Build history of the part. All positions in model axes, mm. A direction names the side the tool comes from. Give positions to 0.01 mm unless a question says otherwise; leave off trailing zeros. Order: outer loops, then holes, each group sorted by start corner. A loop starts at its lowest first (then second) coordinate and runs counter-clockwise, first axis right, second up. Notation, with made-up numbers: (-10, 54.25) - (18, 54.25) arc R26 ccw to (18, 79.25) - close; hole circle Ø11 at (84, 35). An arc over 180 degrees is marked (long way). Write each question's results on one line, items separated by ' | '. Start each with the question number.
1) Cut at B-B on z = 12. List the corners of the cut face in (x, y), plus the area to 3 significant figures.
2) Drop flat-ended pins along their axis: pin 1 Ø6 at (y, z) = (-7, 20) entering from -X; pin 2 Ø6 at (x, y) = (9.5, -5.5) entering from +Z; pin 3 Ø0.7 at (x, z) = (-13, 28) entering from +Y; pin 4 Ø3 at (y, z) = (4, 13) entering from +X. Give the stop position or say it passes through.
3) Drill centre lines: line 1 along Y through (x, z) = (0, 10); line 2 along Z through (x, y) = (11.75, 3.75); line 3 along Z through (x, y) = (12, -7.5). Where is each one in solid material? Low to high. Write a range as from..to.
4) Tool access for faces 1 (the face through (-10.25, 9.09, 29.45)), 2 (the face through (-13, 0, 28)), 3 (the face through (-12, -2, 26)): list every direction of +Z, -Z, +X, -X, +Y, -Y with a clear straight run to the whole face (end or side of a thin tool).
5) Cut at A-A on x = 0. List the corners of the cut face in (y, z), plus the area to 3 significant figures.
6) Two-plate mould, pull along Z, no slides. Class faces 4 (the face through (10.43, -8.88, 29.45)), 5 (the face through (9.5, -8.1, 26.9)), 6 (the face through (10.526, -8.966, 27.131)): +Z half, -Z half, draft (parallel to the pull), parting line (faces both ways), or undercut.
from build123d import *

# Parameters (mm, degrees)
IZIM1_R                     = 15
IZIM1_R_2                   = 13.5
Y_KSEKLIK_EKSTR_ZYON1_DEPTH = 30
Y_KSEKLIK_EKSTR_ZYON2_START = -4
IZIM3_R                     = 13.5
IZIM3_R_2                   = 12
Y_KSEKLIK_EKSTR_ZYON2_DEPTH = 4


with BuildPart() as part:
    # Çizim1 → Yükseklik-Ekstrüzyon1 (new body)
    with BuildSketch(Plane.XY):
        Circle(IZIM1_R)
        Circle(IZIM1_R_2, mode=Mode.SUBTRACT)
    extrude(amount=Y_KSEKLIK_EKSTR_ZYON1_DEPTH)

    # Çizim3 → Yükseklik-Ekstrüzyon2 (add)
    with BuildSketch(Plane.XY.offset(30).offset(Y_KSEKLIK_EKSTR_ZYON2_START)):
        Circle(IZIM3_R)
        Circle(IZIM3_R_2, mode=Mode.SUBTRACT)
    extrude(amount=Y_KSEKLIK_EKSTR_ZYON2_DEPTH)

    # Kes-Süpür2: sweep along a path in Çizim5
    with BuildLine(Plane.XY.offset(30)) as kes_s_p_r2_path:
        ThreePointArc((-1.906671483, 13.566672542), (-10.339521249, 8.988008697), (-13.7, 0))
    # Çizim4 → Kes-Süpür2 (sweep, cut)
    with BuildSketch(Plane(origin=(0, 0, 0), x_dir=(1, 0, 0), z_dir=(0, 1, 0))):
        Polygon((-13.7, -30), (-13.7, -28.88), (-14.43, -28.23), (-13.7, -26.9), (-11.7, -26.9), (-11.7, -30), align=None)
    kes_s_p_r2 = sweep(path=kes_s_p_r2_path.line, mode=Mode.SUBTRACT)

    # Aynalama2: Kes-Süpür2 across plane
    add(kes_s_p_r2.mirror(Plane(origin=(0, 0, 0), x_dir=(0, 0, 1), z_dir=(0.7547095802227689, -0.6560590289905109, 0))), mode=Mode.SUBTRACT)


solid = part.part
Results:
1) outline: circle Ø30 at (0, 0); hole circle Ø27 at (0, 0) | area: 134 mm^2
2) pin 1: x = -14.46 | pin 2: z = 30 | pin 3: y = 8.06 | pin 4: x = 14.79
3) line 1: -15..-13.5, 13.5..15 | line 2: 26..30 | line 3: 0..27.72, 28.48..30
4) face 1: +Z | face 2: none | face 3: -Z
5) outline: (-15, 0) - (-13.5, 0) - (-13.5, 26) - (-12, 26) - (-12, 30) - (-15, 30) - close; (12, 26) - (13.5, 26) - (13.5, 0) - (15, 0) - (15, 30) - (12, 30) - close | area: 102 mm^2
6) face 4: draft | face 5: +Z half | face 6: undercut
